Autodesk Inventor part; units mm, degrees
ref_plane "YZ Plane" through (0, 0, 0) normal (1, 0, 0) x (0, 1, 0)
ref_plane "XZ Plane" through (0, 0, 0) normal (0, 1, 0) x (-1, 0, 0)
ref_plane "XY Plane" through (0, 0, 0) normal (0, 0, 1) x (1, 0, 0)
sketch "Sketch1" plane through (0, 0, 0) normal (0, 0, 1) x (1, 0, 0)
  line L0 (0, 0) -> (25, 0)
  line L1 (25, 0) -> (25, 25)
  line L2 (25, 25) -> (0, 25)
  line L3 (0, 25) -> (0, 0)
  line L4 (3, 22) -> (22, 22)
  line L5 (22, 22) -> (22, 3)
  line L6 (22, 3) -> (3, 3)
  line L7 (3, 3) -> (3, 22)
  dimension "d0" = 25
  dimension "d1" = 25
  dimension "d2" = 3
extrude "Extrusion1" add sketch "Sketch1" along normal blind 525
sketch "Sketch2" plane through (25, 0, 0) normal (1, 0, 0) x (0, 0, -1)
  line L0 (0, 0) -> (0, 25)
  line L1 (0, 25) -> (-525, 25)
  line L2 (-525, 0) -> (-525, 25)
  line L3 (0, 0) -> (-525, 0)
  line L4 (-525, 25) -> (-500, 0)
  line L5 (-525, 25) -> (-489.6447, 25) construction
  line L6 (0, 25) -> (-25, 0)
  line L7 (0, 25) -> (35.3553, 25) construction
  dimension "d5" = 45
  dimension "d6" = 135
extrude "Extrusion2" cut sketch "Sketch2" against normal blind 500 contours L3 L6 L0 | L4 L3 L2
sketch "Sketch3" plane through (25, 25, 525) normal (1, 0, 0) x (0, 0, -1)
  line L0 (500, -25) -> (25, -25)
  line L1 (525, 0) -> (0, 0)
  line L2 (25, -25) -> (0, 0)
  point P0 (525, -25)
  point P1 (55, -12.5)
  point P2 (495, -12.5)
  point P3 (262.5, 0)
  point P4 (12.5, -12.5)
  point P5 (12.5, -12.5)
  dimension "d9" = 440
  dimension "d10" = 12.5
  dimension "d50" = 42.5
hole "Hole1" at (25, 12.5, 30) direction (-1, 0, 0) diameter 12 depth 8 tip angle 118
sketch "Sketch5" plane through (0, 25, 0) normal (-1, 0, 0) x (0, 0, 1)
  circle A0 centre (30, -12.5) radius 6
  line L0 (0, 0) -> (525, 0)
  line L1 (457.5, 0) -> (482.5, 0)
  line L2 (482.5, 0) -> (482.5, -22)
  line L3 (482.5, -22) -> (457.5, -22)
  line L4 (457.5, -22) -> (457.5, 0)
  circle A1 centre (30, -12.5) radius 4.5
  point P0 (0, -25)
  point P1 (470, -12.5)
  point P2 (470, 0)
  dimension "d33" = 440
  dimension "d51" = 12.5
  dimension "d52" = 25
  dimension "d53" = 22
  dimension "d54" = 0
  dimension "d57" = 9
extrude "Extrusion3" cut sketch "Sketch5" against normal through all contours L0 L2 L3 L4 | A1
properties part number "P402" material "Aluminum 6061"
Geometry check sheet. Reference: the model listing, model coordinates, mm. A direction names the side the tool comes from. Coordinates: 2 decimals unless noted, no trailing zeros. Write each loop counter-clockwise with the first axis right and the second up, starting at its lowest first coordinate (ties: lowest second). Pieces come first, ordered by that corner, then holes. Notation, with made-up numbers: M 58,87.25 L 83,87.25 A19 ccw 83,114.25 Z; hole C -13,74 d5. An arc over 180 degrees is marked long. One line per item, written item: value. Start each with the question number.
(1) Sectioned sample at A-A, the plane y = 12.5. Enter the section's corners in (x, z).
(2) Sectioned sample at C-C, the plane x = 15.5. Enter the section's corners in (y, z), and give its area (4 significant figures).
(3) Tool access check on faces 4 (the face through (23.48, 8.44, 34.42)), 5 (the face through (12, 22, 502)), 6 (the face through (12, 23, 457.5)). Record the directions out of +Z, -Z, +X, -X, +Y, -Y that give a thin tool (end or side, any length) a straight path to the whole face; none if there is none.
(4) Sectioned sample at B-B, the plane z = 88.5. Enter the section's corners in (x, y), and give its area (3 significant figures).
(5) Scan lines: line 1 along Y through (x, z) = (2.2, 30); line 2 along X through (y, z) = (9.5, 97); line 3 along Y through (x, z) = (23.3, 30). Record each from-to range of solid material in increasing order. Write a range as [from, to].
(6) Sectioned sample at D-D, the plane z = 30. Enter the section's corners in (x, y), and give its area (3 significant figures).
(7) Release check for a two-part mould opening along Y. For faces 1 (the face through (22, 13, 227)), 2 (the face through (13.4, 22.2, 482.5)), 3 (the face through (24, 13, 513)) record: released by +Y, released by -Y, zero draft, split by the parting line, or undercut.
(8) Depth check by flat-ended pin: pin 1 (11.5 mm diameter, centred on y = 12.5, z = 30, fed in from +X). Enter the tip coordinate at first touch or a pass-through.
Filled sheet:
1. outline: M 0,12.5 L 3,12.5 L 3,25.5 L 0,25.5 Z; M 0,34.5 L 3,34.5 L 3,457.5 L 0,457.5 Z; M 0,482.5 L 3,482.5 L 3,512.5 L 0,512.5 Z; M 22,12.5 L 25,12.5 L 25,24 L 22,24 Z; M 22,36 L 25,36 L 25,457.5 L 22,457.5 Z; M 22,482.5 L 25,482.5 L 25,512.5 L 22,512.5 Z
2. outline: M 0,25 L 3,22 L 3,503 L 0,500 Z; M 22,3 L 25,0 L 25,457.5 L 22,457.5 Z; M 22,482.5 L 25,482.5 L 25,525 L 22,522 Z
2. area: 2,925 mm²
3. face 4: +X
3. face 5: +Z, -Z
3. face 6: +X, -X, +Y
4. outline: M 0,0 L 25,0 L 25,25 L 0,25 Z; hole M 3,3 L 22,3 L 22,22 L 3,22 Z
4. area: 264 mm²
5. line 1: [0, 8], [17, 25]
5. line 2: [0, 3], [22, 25]
5. line 3: [0, 6.5], [18.5, 25]
6. outline: M 0,0 L 25,0 L 25,6.5 L 22,6.5 L 22,3 L 3,3 L 3,8 L 0,8 Z; M 0,17 L 3,17 L 3,22 L 22,22 L 22,18.5 L 25,18.5 L 25,25 L 0,25 Z
6. area: 201 mm²
7. face 1: undercut
7. face 2: zero draft
7. face 3: released by -Y
8. pin 1: x = 3
